```python
from build123d import *

# Parameters (mm, degrees)
SKETCH_R        = 5
PAD_DEPTH       = 35
SKETCH019_R     = 3.5
POCKET007_DEPTH = 8
SKETCH066_R     = 3.2
POCKET_DEPTH    = 3.4
SKETCH067_R     = 3.2
POCKET025_DEPTH = 3.4
SKETCH068_R     = 3.2
POCKET026_DEPTH = 3.4
SKETCH069_R     = 3.2
POCKET027_DEPTH = 3.4


with BuildPart() as part:
    # Sketch → Pad (new body)
    with BuildSketch(Plane.XY):
        Circle(SKETCH_R)
    extrude(amount=PAD_DEPTH)

    # Sketch019 → Pocket007 (cut)
    with BuildSketch(Plane.XY.offset(35)):
        Circle(SKETCH019_R)
    extrude(amount=-POCKET007_DEPTH, mode=Mode.SUBTRACT)

    # Sketch034 → Revolution (revolve)
    with BuildSketch(Plane.XZ):
        with BuildLine():
            ThreePointArc((6.37868, 6.121321), (5.728361, 5.148051), (5.5, 4))
            ThreePointArc((5.5, 4), (5.728361, 2.851949), (6.37868, 1.878679))
            Line((6.37868, 1.878679), (7, 1.25736))
            Line((7, 0), (7, 1.25736))
            Line((0, 0), (7, 0))
            Line((0, 8), (0, 0))
            Line((7, 8), (0, 8))
            Line((7, 6.74264), (7, 8))
            Line((6.37868, 6.121321), (7, 6.74264))
        make_face()
    revolve(axis=Axis((0, 0, 0), (0, 0, 1)))

    # Sketch066 (on DatumPlane) → Pocket (cut)
    with BuildSketch(Plane(origin=(5, 0, 35), x_dir=(0, 1, 0), z_dir=(1, 0, 0))):
        with Locations((0, -12.75)):
            Circle(SKETCH066_R)
    extrude(amount=-POCKET_DEPTH, mode=Mode.SUBTRACT)

    # Sketch067 (on DatumPlane) → Pocket025 (cut)
    with BuildSketch(Plane(origin=(0, 5, 35), x_dir=(-1, 0, 0), z_dir=(0, 1, 0))):
        with Locations((0, -22.25)):
            Circle(SKETCH067_R)
    extrude(amount=-POCKET025_DEPTH, mode=Mode.SUBTRACT)

    # Sketch068 (on DatumPlane) → Pocket026 (cut)
    with BuildSketch(Plane(origin=(-5, 0, 35), x_dir=(0, -1, 0), z_dir=(-1, 0, 0))):
        with Locations((0, -12.75)):
            Circle(SKETCH068_R)
    extrude(amount=-POCKET026_DEPTH, mode=Mode.SUBTRACT)

    # Sketch069 (on DatumPlane) → Pocket027 (cut)
    with BuildSketch(Plane(origin=(0, -5, 35), x_dir=(1, 0, 0), z_dir=(0, -1, 0))):
        with Locations((0, -22.25)):
            Circle(SKETCH069_R)
    extrude(amount=-POCKET027_DEPTH, mode=Mode.SUBTRACT)


solid = part.part
```
Work out the finished part from the listing and answer in its coordinate system (mm). A direction names the side the tool comes from. Coordinates: 2 decimals unless noted, no trailing zeros. Write each loop counter-clockwise with the first axis right and the second up, starting at its lowest first coordinate (ties: lowest second). Pieces come first, ordered by that corner, then holes. Notation, with made-up numbers: (26, 77.25) - (75, 77.25) arc R31 ccw to (75, 102.25) - close; hole circle Ø6 at (-8, 1.25). An arc over 180 degrees is marked (long way). Answer as a JSON object with one key per item and string values.
Q1. Find section D-D (z = 29.5). Write down the section's boundary in (x, y).
Results list:
{"outline": "circle Ø10 at (0, 0); hole circle Ø7 at (0, 0)"}
Q2. Which of the six approach directions +Z, -Z, +X, -X, +Y, -Y give full straight-line access (tool end or side, diameter ignored) to faces 1 (the cylindrical face through (2.946, -3.197, 22.391)), 2 (the flat face through (0, -1.6, 13)), 3 (the cylindrical face through (-3.685, 3.379, 21.311))?
Results list:
{"face 1": "+X", "face 2": "-Y", "face 3": "+Z"}
Q3. Consider L1, parallel to Y at x = 0, z = 32.5; L2, parallel to Z at x = -2.95, y = 0; L3, parallel to Z at x = 0, y = 3.7. Determine where each line is inside the solid, lowest interval first. Write a range as from..to.
Results list:
{"L1": "y = -5..-3.5, 3.5..5", "L2": "z = 0..19.05, 25.45..27", "L3": "z = 0..9.55, 15.95..35"}
Q4. Given pin 1 Ø1.5 at (x, z) = (3, 16.5) entering from -Y; pin 2 Ø1 at (y, z) = (0.5, 5.5) entering from -X; pin 3 Ø3 at (y, z) = (1, 23) entering from +X, each flat-ended and moving along its own axis, determine where each tip first touches the part or whether it passes through.
Results list:
{"pin 1": "stops at y = -4.47", "pin 2": "stops at x = -6.25", "pin 3": "stops at x = 1.6"}
Q5. For a pull along Y with two mould halves and no side action, classify faces 4 (the flat face through (0, 1.6, 13)), 5 (the flat face through (0, 0, 0)), 6 (the cylindrical face through (3.233, -1.341, 31.056)), 7 (the flat face through (-1.6, 0, 22)) as pulls with the +Y half, pulls with the -Y half, needs draft (parallel to the pull), parting line crosses it, or undercut.
Results list:
{"face 4": "pulls with the +Y half", "face 5": "needs draft", "face 6": "undercut", "face 7": "undercut"}
Q6. Find section C-C (z = 12.75). Write down the section's boundary in (x, y), plus the area to 3 significant figures.
Results list:
{"outline": "(-3.2, -3.84) - (-3.2, -1.6) - (3.2, -1.6) - (3.2, -3.84) arc R5 ccw to (3.2, 3.84) - (3.2, 1.6) - (-3.2, 1.6) - (-3.2, 3.84) arc R5 ccw to start", "area": "39.7 mm^2"}
